Print and shaded views of the part. All mm, measured from the part's lowest x, y and z. Round coordinates to 2 decimals unless told otherwise and drop trailing zeros. Loops run counter-clockwise (first coordinate to the right, second up) from the corner with the lowest first, then second, coordinate; pieces in that order, holes last. Notation, with made-up numbers: (55.25, 22.5) -> (107.25, 22.5) arc R18 cw to (107.25, 41.5) -> close; hole circle Ø3 at (19.25, 25.25). An arc over 180 degrees is marked (long way). Use a Markdown table: item, result.
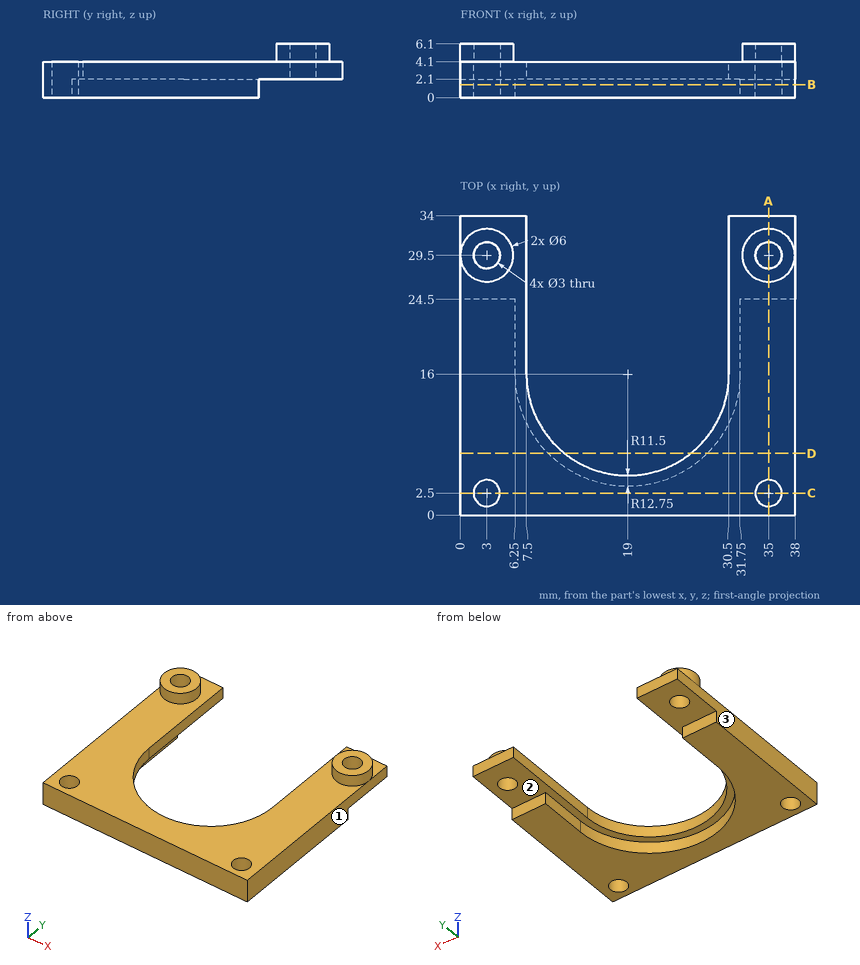
Q1. Band-saw the part on C-C, the plane y = 2.5. Give the cut face in (x, z).
Results list:
| item | result |
|---|---|
| outline | (0, 0) -> (1.5, 0) -> (1.5, 4.1) -> (0, 4.1) -> close; (4.5, 0) -> (33.5, 0) -> (33.5, 4.1) -> (4.5, 4.1) -> close; (36.5, 0) -> (38, 0) -> (38, 4.1) -> (36.5, 4.1) -> close |
Q2. Band-saw the part on D-D, the plane y = 7. Give the cut face in (x, z).
Results list:
| item | result |
|---|---|
| outline | (0, 0) -> (9.97, 0) -> (9.97, 2.1) -> (11.84, 2.1) -> (11.84, 4.1) -> (0, 4.1) -> close; (26.16, 2.1) -> (28.03, 2.1) -> (28.03, 0) -> (38, 0) -> (38, 4.1) -> (26.16, 4.1) -> close |
Q3. Drill centre lines: L1, parallel to Y at x = 35, z = 3.05; L2, parallel to X at y = 29.5, z = 3.45; L3, parallel to X at y = 23.5, z = 2.5. Where is each one in solid material? Low to high. Write a range as from..to.
Results list:
| item | result |
|---|---|
| L1 | y = 0..1, 4..28, 31..34 |
| L2 | x = 0..1.5, 4.5..7.5, 30.5..33.5, 36.5..38 |
| L3 | x = 0..7.5, 30.5..38 |
Q4. Pull direction X, two halves, no side cores. Call the marked faces 1, 2 and 3: released by +X, released by -X, zero draft, split by the parting line, or undercut.
Results list:
| item | result |
|---|---|
| face 1 | released by +X |
| face 2 | undercut |
| face 3 | released by -X |
Q5. Band-saw the part on B-B, the plane z = 1.5. Give the cut face in (x, y), plus the area to 3 significant figures.
Results list:
| item | result |
|---|---|
| outline | (0, 0) -> (38, 0) -> (38, 24.5) -> (31.75, 24.5) -> (31.75, 16) arc R12.75 cw to (6.25, 16) -> (6.25, 24.5) -> (0, 24.5) -> close; hole circle Ø3 at (3, 2.5); hole circle Ø3 at (35, 2.5) |
| area | 445 mm² |
Q6. Band-saw the part on A-A, the plane x = 35. Give the cut face in (y, z).
Results list:
| item | result |
|---|---|
| outline | (0, 0) -> (1, 0) -> (1, 4.1) -> (0, 4.1) -> close; (4, 0) -> (24.5, 0) -> (24.5, 2.1) -> (28, 2.1) -> (28, 6.1) -> (26.5, 6.1) -> (26.5, 4.1) -> (4, 4.1) -> close; (31, 2.1) -> (34, 2.1) -> (34, 4.1) -> (32.5, 4.1) -> (32.5, 6.1) -> (31, 6.1) -> close |
Q7. Flat gauge pins, fed straight in: pin 1 (12 mm diameter, centred on x = 28.5, y = 13.5, fed in from +Z); pin 2 (4 mm diameter, centred on x = 14, y = 9, fed in from -Z); pin 3 (0.6 mm diameter, centred on x = 2.5, z = 1, fed in from +Y); pin 4 (4 mm diameter, centred on x = 3, y = 29.5, fed in from -Z). Where does each tip first touch, or does it go through?
Results list:
| item | result |
|---|---|
| pin 1 | stops at z = 4.1 |
| pin 2 | passes through |
| pin 3 | stops at y = 24.5 |
| pin 4 | stops at z = 2.1 |
